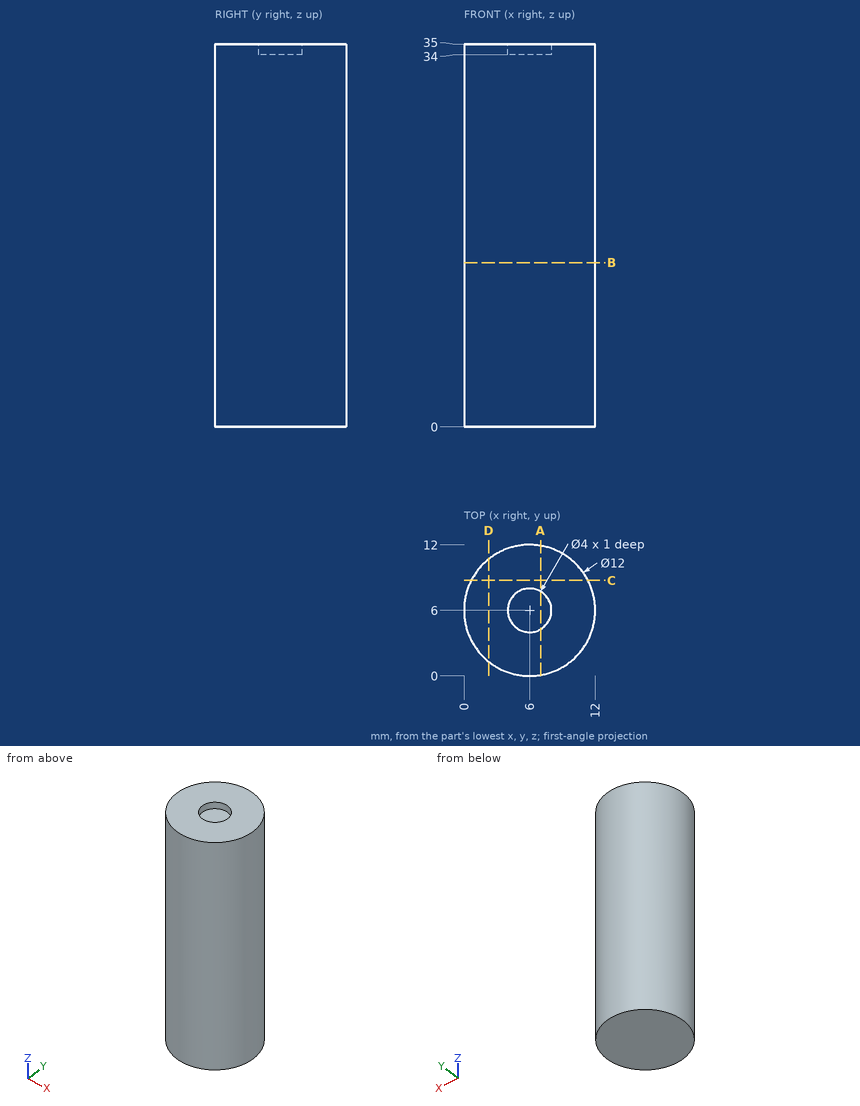
For this review, use the dimensioned drawing (mm, ordinates from the lowest corner) and the shaded views. Coordinates: 2 decimals unless noted, no trailing zeros. Loops run counter-clockwise (first coordinate to the right, second up) from the corner with the lowest first, then second, coordinate; pieces in that order, holes last. Notation, with made-up numbers: (-9.5, -14) -> (39.5, -14) arc R12 cw to (39.5, 7) -> close; hole circle Ø6 at (9.25, 27). An arc over 180 degrees is marked (long way). Return JSON: item names as keys, results as strings. Group by question number.
(1) For pin 1 Ø4 at (x, z) = (2, 4.5) entering from -Y; pin 2 Ø1.2 at (x, y) = (5.5, 6) entering from +Z; pin 3 Ø1 at (x, z) = (2.5, 21.5) entering from -Y, all flat-tipped, find the tip position at first contact; note any pin that passes through.
(2) Consider section B-B, the plane z = 15. Give the boundary of the cut face in (x, y), plus the area to 3 significant figures.
(3) Consider section A-A, the plane x = 7. Give the boundary of the cut face in (y, z), plus the area to 3 significant figures.
(4) Consider section D-D, the plane x = 2.25. Give the boundary of the cut face in (y, z).
(5) To check wall thickness, follow L1, parallel to Y at x = 6, z = 34.35; L2, parallel to Z at x = 6.5, y = 4.5; L3, parallel to Y at x = 5, z = 33. State the ranges of each line that lie inside material, in increasing order.
(6) Consider section C-C, the plane y = 8.75. Give the boundary of the cut face in (x, z).
Results below:
{
 "1": {"pin 1": "stops at y = 0.34", "pin 2": "stops at z = 34", "pin 3": "stops at y = 0.8"},
 "2": {"outline": "circle Ø12 at (6, 6)", "area": "113 mm2"},
 "3": {"outline": "(0.08, 0) -> (11.92, 0) -> (11.92, 35) -> (7.73, 35) -> (7.73, 34) -> (4.27, 34) -> (4.27, 35) -> (0.08, 35) -> close", "area": "411 mm2"},
 "4": {"outline": "(1.32, 0) -> (10.68, 0) -> (10.68, 35) -> (1.32, 35) -> close"},
 "5": {"L1": "y = 0 to 4, 8 to 12", "L2": "z = 0 to 34", "L3": "y = 0.08 to 11.92"},
 "6": {"outline": "(0.67, 0) -> (11.33, 0) -> (11.33, 35) -> (0.67, 35) -> close"}
}
